Verification items for this drawing (mm, ordinates from the low corner). Round coordinates to 2 decimals unless told otherwise and drop trailing zeros. Loops run counter-clockwise (first coordinate to the right, second up) from the corner with the lowest first, then second, coordinate; pieces in that order, holes last. Notation, with made-up numbers: (-35, 77.5) - (-8, 77.5) arc R22 cw to (-8, 103.5) - close; hole circle Ø2 at (75, -5.5). An arc over 180 degrees is marked (long way). Write item = value, one per line.
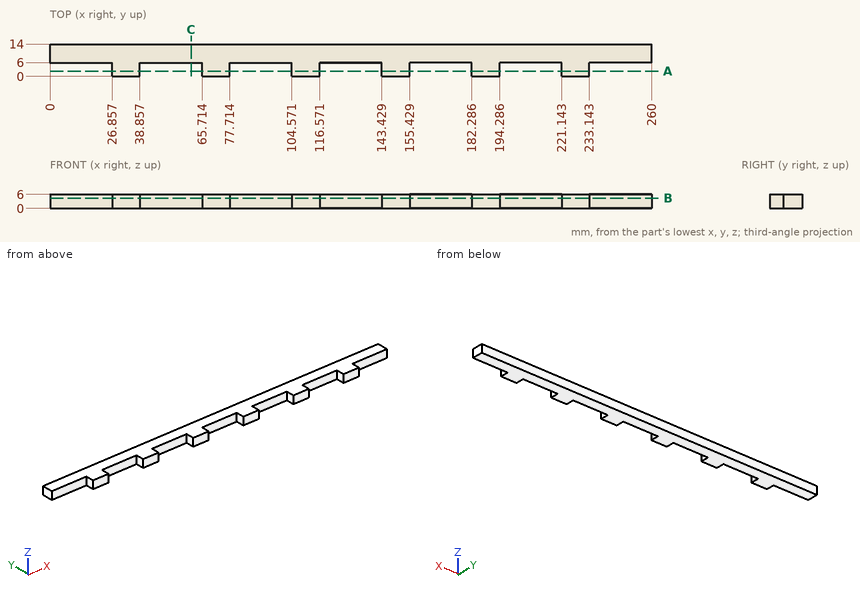
(1) Section check B-B (z = 4.4). Enter the section's corners in (x, y) (1 decimal), then the cut area to 3 significant figures.
Answers follow:
outline = (0, 6) - (26.9, 6) - (26.9, 0) - (38.9, 0) - (38.9, 6) - (65.7, 6) - (65.7, 0) - (77.7, 0) - (77.7, 6) - (104.6, 6) - (104.6, 0) - (116.6, 0) - (116.6, 6) - (143.4, 6) - (143.4, 0) - (155.4, 0) - (155.4, 6) - (182.3, 6) - (182.3, 0) - (194.3, 0) - (194.3, 6) - (221.1, 6) - (221.1, 0) - (233.1, 0) - (233.1, 6) - (260, 6) - (260, 14) - (0, 14) - close
area = 2,510 mm²
(2) Gauge pin test, flat ends, axial feed: pin 1 (1.8 mm diameter, centred on x = 126.5, z = 3, fed in from -Y); pin 2 (1.8 mm diameter, centred on y = 2, z = 4, fed in from +X); pin 3 (3 mm diameter, centred on y = 2, z = 3, fed in from -X). Record the tip position at first contact, or that the pin passes through.
Answers follow:
pin_1 = 6
pin_2 = 233.14
pin_3 = 26.86
(3) Section check C-C (x = 61). Enter the section's corners in (y, z).
Answers follow:
outline = (6, 0) - (14, 0) - (14, 6) - (6, 6) - close
(4) Section check A-A (y = 2.25). Enter the section's corners in (x, z) (1 decimal).
Answers follow:
outline = (26.9, 0) - (38.9, 0) - (38.9, 6) - (26.9, 6) - close; (65.7, 0) - (77.7, 0) - (77.7, 6) - (65.7, 6) - close; (104.6, 0) - (116.6, 0) - (116.6, 6) - (104.6, 6) - close; (143.4, 0) - (155.4, 0) - (155.4, 6) - (143.4, 6) - close; (182.3, 0) - (194.3, 0) - (194.3, 6) - (182.3, 6) - close; (221.1, 0) - (233.1, 0) - (233.1, 6) - (221.1, 6) - close
(5) Scan lines: L1, parallel to X at y = 1, z = 4.65 (1 decimal); L2, parallel to Y at x = 131.5, z = 2.9. Record each from-to range of solid material in increasing order. Write a range as [from, to].
Answers follow:
L1 = [26.9, 38.9], [65.7, 77.7], [104.6, 116.6], [143.4, 155.4], [182.3, 194.3], [221.1, 233.1]
L2 = [6, 14]
